Build history of the part. All positions in model axes, mm. A direction names the side the tool comes from. Round coordinates to 2 decimals unless told otherwise and drop trailing zeros. Write each loop counter-clockwise with the first axis right and the second up, starting at its lowest first coordinate (ties: lowest second). Pieces come first, ordered by that corner, then holes. Notation, with made-up numbers: (-35, -26.75) -> (-21, -26.75) arc R16 ccw to (-21, -5.75) -> close; hole circle Ø1 at (-7, 77). An arc over 180 degrees is marked (long way). Answer in a Markdown table with one row per item.
```python
from build123d import *

# Parameters (mm, degrees)
SKETCH1_R           = 16.65
BOSS_EXTRUDE1_DEPTH = 4.7
SKETCH2_R           = 11.325
BOSS_EXTRUDE2_DEPTH = 4.85
SKETCH3_R           = 14
BOSS_EXTRUDE3_DEPTH = 33.3
FILLET1_R           = 4
CHAMFER1_SIZE       = 1
CHAMFER1_SIZE2      = 11
FILLET2_R           = 1


with BuildPart() as part:
    # Sketch1 → Boss-Extrude1 (new body)
    with BuildSketch(Plane(origin=(0, 0, 0), x_dir=(1, 0, 0), z_dir=(0, 1, 0))):
        with Locations(Location((0, 0, 0), (0, 0, 270))):
            Circle(SKETCH1_R)
    extrude(amount=BOSS_EXTRUDE1_DEPTH)

    # Sketch2 → Boss-Extrude2 (add)
    with BuildSketch(Plane(origin=(0, 4.7, 0), x_dir=(1, 0, 0), z_dir=(0, 1, 0))):
        with Locations(Location((0, 0, 0), (0, 0, 270))):
            Circle(SKETCH2_R)
    extrude(amount=BOSS_EXTRUDE2_DEPTH)

    # Sketch3 → Boss-Extrude3 (add)
    with BuildSketch(Plane.XZ):
        with Locations(Location((0, 0, 0), (0, 0, 270))):
            Circle(SKETCH3_R)
    extrude(amount=BOSS_EXTRUDE3_DEPTH)

    # Fillet1
    fillet1_edges = [part.edges().sort_by_distance(p)[0] for p in [
        (0, 4.7, -16.65),
    ]]
    fillet(fillet1_edges, radius=FILLET1_R)

    # Chamfer1
    chamfer1_edges = [part.edges().sort_by_distance(p)[0] for p in [
        (0, 9.55, -11.325),
    ]]
    chamfer1_side = [part.faces().sort_by_distance(p)[0] for p in [
        (0, 7.125, -11.325),
    ]]
    chamfer(chamfer1_edges, length=CHAMFER1_SIZE, length2=CHAMFER1_SIZE2, reference=chamfer1_side[0])

    # Fillet2
    fillet2_edges = [part.edges().sort_by_distance(p)[0] for p in [
        (0, 8.55, -11.325),
    ]]
    fillet(fillet2_edges, radius=FILLET2_R)


solid = part.part
```
Q1. Wall check: line 1 (X direction, y = -22, z = -6); line 2 (Y direction, x = -1, z = -12); line 3 (Z direction, x = -2, y = -15). Give the ranges that are in metal, low to high. Write a range as [from, to].
A:
| item | result |
|---|---|
| line 1 | [-12.65, 12.65] |
| line 2 | [-33.3, 4.7] |
| line 3 | [-13.86, 13.86] |
Q2. Saw through at A-A on y = -4.5. Write the cut outline in (x, z), plus the area to 3 significant figures.
A:
| item | result |
|---|---|
| outline | circle Ø28 at (0, 0) |
| area | 616 mm² |
Q3. Which spindle directions (+Z, -Z, +X, -X, +Y, -Y) get a long thin tool onto all of the face, cutting with end or side? Do faces 1 (the flat face through (14, 0, -4)), 2 (the flat face through (-11.2, 4.7, -2.9)), 3 (the flat face through (0, -33.3, 0)). Say none if no direction does.
A:
| item | result |
|---|---|
| face 1 | -Y |
| face 2 | +Y |
| face 3 | +Z, -Z, +X, -X, -Y |
Q4. Saw through at B-B on y = 2. Write the cut outline in (x, z), plus the area to 3 significant figures.
A:
| item | result |
|---|---|
| outline | circle Ø32.87 at (0, 0) |
| area | 848 mm² |
Q5. Drop flat-ended pins along their axis: P1, Ø12, axis at y = -19.5, z = -1, coming from the +X side; P2, Ø6, axis at x = 3, y = 2, coming from the +Z side; P3, Ø6, axis at y = -23, z = 5, coming from the +X side. Give the stop position or say it passes through.
A:
| item | result |
|---|---|
| P1 | x = 14 |
| P2 | z = 16.65 |
| P3 | x = 13.86 |
